Build history of the part. All positions in model axes, mm. A direction names the side the tool comes from. Round coordinates to 2 decimals unless told otherwise and drop trailing zeros. Order: outer loops, then holes, each group sorted by start corner. A loop starts at its lowest first (then second) coordinate and runs counter-clockwise, first axis right, second up. Notation, with made-up numbers: (24.25, -6) -> (71.25, -6) arc R18 cw to (71.25, 2) -> close; hole circle Ø8 at (-13.75, -8). An arc over 180 degrees is marked (long way). Write item = value, one per line.
from build123d import *

# Parameters (mm, degrees)
PAD_DEPTH    = 2
POCKET_DEPTH = 7
FILLET004_R  = 1
FILLET005_R  = 0.25


with BuildPart() as arms:
    # Sketch → Pad (new body)
    with BuildSketch(Plane.XY):
        Polygon((-10.055, 1.35), (-10.055, -1.35), (-1.35, -1.35), (-1.35, -10.055), (1.35, -10.055), (1.35, -1.35), (10.055, -1.35), (10.055, 1.35), (1.35, 1.35), (1.35, 10.055), (-1.35, 10.055), (-1.35, 1.35), align=None)
    extrude(amount=PAD_DEPTH)


with BuildPart() as rotation_center_ball:
    # Sketch001 → Revolution (revolve)
    with BuildSketch(Plane.XZ):
        with BuildLine():
            Line((5.5, 2), (5.5, 0))
            Line((5.5, 0), (0, 0))
            Line((0, 8.5), (0, 0))
            Line((3.162278, 8.5), (0, 8.5))
            Line((3.162278, 6.5), (3.162278, 8.5))
            ThreePointArc((5.5, 2), (4.880703, 4.535495), (3.162278, 6.5))
        make_face()
    revolve(axis=Axis((0, 0, 0), (0, 0, 1)))

    # Boolean: union Arms
    add(arms.part)

    # Sketch002 (on ShapeBinder) → Pocket (cut)
    with BuildSketch(Plane(origin=(0, 0, 8.5), x_dir=(-1, 0, 0), z_dir=(0, 0, 1))):
        Polygon((-2.25, 1), (-1, 1), (-1, 2.25), (1, 2.25), (1, 1), (2.25, 1), (2.25, -1), (1, -1), (1, -2.25), (-1, -2.25), (-1, -1), (-2.25, -1), align=None)
    extrude(amount=-POCKET_DEPTH, mode=Mode.SUBTRACT)

    # Fillet004
    fillet004_edges = [rotation_center_ball.edges().sort_by_distance(p)[0] for p in [
        (0, 10.055, 2),
        (10.055, 0, 2),
        (-10.055, 0, 2),
        (0, -10.055, 2),
        (-7.693372, -1.35, 2),
        (-7.693372, 1.35, 2),
        (-1.35, -7.693372, 2),
        (1.35, -7.693372, 2),
        (7.693372, -1.35, 2),
        (7.693372, 1.35, 2),
        (-1.35, 7.693372, 2),
        (1.35, 7.693372, 2),
    ]]
    fillet(fillet004_edges, radius=FILLET004_R)

    # Fillet005
    fillet005_edges = [rotation_center_ball.edges().sort_by_distance(p)[0] for p in [
        (-3.162278, 0, 8.5),
    ]]
    fillet(fillet005_edges, radius=FILLET005_R)


solid = rotation_center_ball.part
Q1. Flat gauge pins, fed straight in: pin 1 (1.5 mm diameter, centred on x = 2, z = 5, fed in from +Y); pin 2 (0.8 mm diameter, centred on y = -8, z = 0.5, fed in from +X); pin 3 (1 mm diameter, centred on x = 4.5, y = -5.5, fed in from -Z); pin 4 (0.6 mm diameter, centred on x = 0, y = -7, fed in from +Z). Where does each tip first touch, or does it go through?
Check values:
pin_1 = 4.7
pin_2 = 1.35
pin_3 = through
pin_4 = 2
Q2. Probe probe 1 along X at (y, z) = (-1.75, 1.75); probe 2 along Y at (x, z) = (1.75, 4.5); probe 3 along Y at (x, z) = (-0.75, 7.5). List the from-to ranges inside material, lowest first.
Check values:
probe_1 = -5.21 to -1, 1 to 5.21
probe_2 = -4.58 to -1, 1 to 4.58
probe_3 = -3.07 to -2.25, 2.25 to 3.07
Q3. Which spindle directions (+Z, -Z, +X, -X, +Y, -Y) get a long thin tool onto all of the face, cutting with end or side? Do faces 1 (the face through (-7.66, -1.065, 1.699)), 2 (the face through (1, -2, 5)), 3 (the face through (7.66, 1.065, 1.699)). Say none if no direction does.
Check values:
face_1 = +Z, -X, -Y
face_2 = +Z
face_3 = +Z, +X, +Y
Q4. Mould opens along X. For faces 4 (the face through (0, 0, 1.5)), 5 (the face through (-1.065, -7.726, 1.699)), 6 (the face through (3.93, 3.85, 0.99)) say: released by +X, released by -X, zero draft, split by the parting line, or undercut.
Check values:
face_4 = undercut
face_5 = released by -X
face_6 = released by +X
Q5. Cut at A-A, the plane y = -8.5. List the corners of the cut face in (x, z), and give its area (3 significant figures).
Check values:
outline = (-1.35, 0) -> (1.35, 0) -> (1.35, 1) arc R1 ccw to (0.35, 2) -> (-0.35, 2) arc R1 ccw to (-1.35, 1) -> close
area = 4.97 mm²
